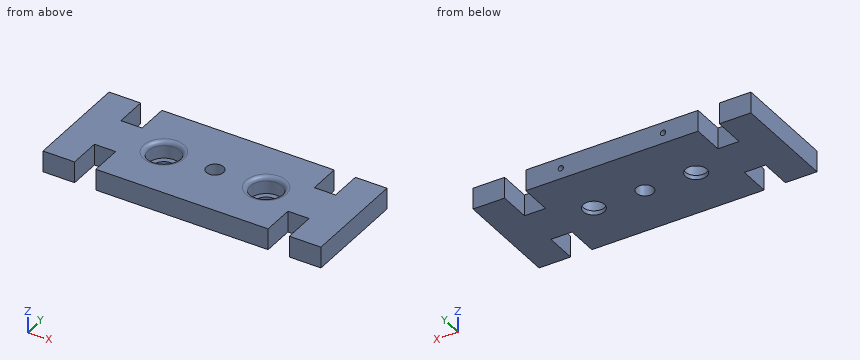
Autodesk Inventor part; units mm, degrees
ref_plane "YZ Plane" through (0, 0, 0) normal (1, 0, 0) x (0, 1, 0)
ref_plane "XZ Plane" through (0, 0, 0) normal (0, 1, 0) x (-1, 0, 0)
ref_plane "XY Plane" through (0, 0, 0) normal (0, 0, 1) x (1, 0, 0)
sketch "Sketch1" plane through (0, 0, 0) normal (0, 0, 1) x (1, 0, 0)
  line L0 (65.5, 25) -> (-65.5, 25)
  line L1 (-65.5, 25) -> (-65.5, -25)
  line L2 (-65.5, -25) -> (65.5, -25)
  line L3 (65.5, -25) -> (65.5, 25)
  line L4 (-40.6, 25) -> (-40.6, 10)
  line L5 (-40.6, 10) -> (-50.6, 10)
  line L6 (-50.6, 10) -> (-50.6, 25)
  line L7 (-40.6, -25) -> (-40.6, -10)
  line L8 (-40.6, -10) -> (-50.6, -10)
  line L9 (-50.6, -10) -> (-50.6, -25)
  line L10 (40.6, 25) -> (40.6, 10)
  line L11 (40.6, 10) -> (50.6, 10)
  line L12 (50.6, 10) -> (50.6, 25)
  line L13 (40.6, -25) -> (40.6, -10)
  line L14 (40.6, -10) -> (50.6, -10)
  line L15 (50.6, -10) -> (50.6, -25)
  circle A0 centre (24.1, 0) radius 7.5
  circle A1 centre (-24.1, 0) radius 7.5
  circle A2 centre (24.1, 0) radius 7.5
  circle A3 centre (-24.1, 0) radius 7.5
  circle A4 centre (0, 0) radius 4
  dimension "d0" = 15
  dimension "d1" = 15
  dimension "d2" = 15
  dimension "d3" = 15
  dimension "d8" = 15
  dimension "d9" = 15
  dimension "d30" = 8
extrude "Extrusion2" add sketch "Sketch1" along normal blind 10 contours L3 L2 L15 L14 L13 L7 L8 L9 L1 L0 L6 L5 L4 L10 L11 L12 | A4
sketch "Sketch2" plane through (-40.6, 25, 0) normal (0, 1, 0) x (1, 0, 0)
  circle A0 centre (64.7, -5) radius 1.25
  circle A1 centre (16.5, -5) radius 1.25
  point P0 (40.6, 0)
  dimension "d15" = 2.5
  dimension "d16" = 2.5
extrude "Extrusion3" cut sketch "Sketch2" against normal blind 10
sketch "Sketch3" plane through (0, 0, 0) normal (0, 0, -1) x (-1, 0, 0)
  circle A0 centre (0, 0) radius 24.1
  circle A1 centre (-24.1, 0) radius 5
  circle A2 centre (24.1, 0) radius 5
  circle A3 centre (-24.1, 0) radius 7.5
  circle A4 centre (24.1, 0) radius 7.5
  dimension "d25" = 48.2
  dimension "d26" = 10
  dimension "d27" = 10
extrude "Extrusion6" add sketch "Sketch3" against normal blind 2 contours A2 A0 A4 | A0 A4 A2 | A3 A0 A1 | A0 A1 A3
extrude "Extrusion7" cut sketch "Sketch1" along normal blind 10 contours A4
fillet "Fillet1" radius 2 2 edges at (-31.6, 0, 10) (16.6, 0, 10)
properties part number "prepazka-sablona"
For this review, take the finished solid that the model builds, in its own axes (mm). Round coordinates to 2 decimals unless told otherwise and drop trailing zeros. Order: outer loops, then holes, each group sorted by start corner. A loop starts at its lowest first (then second) coordinate and runs counter-clockwise, first axis right, second up. Notation, with made-up numbers: M 83.25,37 L 132.25,37 A15 ccw 132.25,53 Z; hole C 77.25,67.25 d2. An arc over 180 degrees is marked long. Write each question's results on one line, items separated by ' | '. Start each with the question number.
1. Add section B-B (y = 0). State the section outline as (x, z) points, then the cut area to 3 significant figures.
2. To check wall thickness, follow L1, parallel to X at y = 21, z = 5; L2, parallel to X at y = 13.5, z = 7.5; L3, parallel to Y at x = 24.1, z = 1.3. State the ranges of each line that lie inside material, in increasing order. Write a range as [from, to].
3. Add section D-D (x = 0). State the section outline as (y, z) points.
4. Clearance check with flat-ended pins moving along their axes: pin 1 Ø13.5 at (x, y) = (24.1, 0) entering from -Z; pin 2 Ø12 at (x, y) = (22, -1) entering from +Z; pin 3 Ø1.2 at (x, z) = (24, 5.5) entering from +Y. State where each tip first meets the part, or that it passes through.
5. Add section C-C (y = 13). State the section outline as (x, z) points.
6. Add section A-A (x = 24.1). State the section outline as (y, z) points.
Output values:
1) outline: M -65.5,0 L -29.1,0 L -29.1,2 L -31.6,2 L -31.6,8 A2 ccw -33.6,10 L -65.5,10 Z; M -19.1,0 L -4,0 L -4,10 L -14.6,10 A2 ccw -16.6,8 L -16.6,2 L -19.1,2 Z; M 4,0 L 19.1,0 L 19.1,2 L 16.6,2 L 16.6,8 A2 ccw 14.6,10 L 4,10 Z; M 29.1,0 L 65.5,0 L 65.5,10 L 33.6,10 A2 ccw 31.6,8 L 31.6,2 L 29.1,2 Z | area: 947 mm^2
2) L1: [-65.5, -50.6], [-40.6, -25.35], [-22.85, 22.85], [25.35, 40.6], [50.6, 65.5] | L2: [-65.5, -50.6], [-40.6, 40.6], [50.6, 65.5] | L3: [-25, -5], [5, 25]
3) outline: M -25,0 L -4,0 L -4,10 L -25,10 Z; M 4,0 L 25,0 L 25,10 L 4,10 Z
4) pin 1: z = 0 | pin 2: z = 9.62 | pin 3: y = 15
5) outline: M -65.5,0 L -50.6,0 L -50.6,10 L -65.5,10 Z; M -40.6,0 L 40.6,0 L 40.6,10 L -40.6,10 Z; M 50.6,0 L 65.5,0 L 65.5,10 L 50.6,10 Z
6) outline: M -25,0 L -5,0 L -5,2 L -7.5,2 L -7.5,8 A2 ccw -9.5,10 L -25,10 Z; M 5,0 L 25,0 L 25,3.75 L 15,3.75 L 15,6.25 L 25,6.25 L 25,10 L 9.5,10 A2 ccw 7.5,8 L 7.5,2 L 5,2 Z
